from build123d import *

# Parameters (mm, degrees)
F1_DEPTH = 15
F3_DEPTH = 2.4
F4_R     = 1.8
F5_DEPTH = 13.301
F7_D     = 4


with BuildPart() as f1:
    # F0 (on Front) → F1 (new body)
    with BuildSketch(Plane.XZ):
        with BuildLine():
            Line((40, 0), (0, 0))
            Line((0, 0), (0, -3))
            Line((0, -3), (40, -3))
            ThreePointArc((40, -3), (47.202138, 7.972773), (34.269901, 10.215488))
            ThreePointArc((34.269901, 10.215488), (31.944896, 8.577711), (29.160258, 8))
            Line((29.160258, 8), (13, 8))
            Line((13, 8), (13, 5))
            Line((13, 5), (29.160258, 5))
            ThreePointArc((29.160258, 5), (33.138313, 5.825302), (36.459748, 8.164983))
            ThreePointArc((36.459748, 8.164983), (44.449729, 6.779356), (40, 0))
        make_face()
    extrude(amount=F1_DEPTH)

    # F2 (on face) → F3 (cut)
    with BuildSketch(Plane(origin=(0, 0, -3), x_dir=(1, 0, 0), z_dir=(0, 0, -1))):
        Polygon((21.645448, 10.35), (18.354552, 10.35), (16.709103, 7.5), (18.354552, 4.65), (21.645448, 4.65), (23.290897, 7.5), align=None)
    extrude(amount=-F3_DEPTH, mode=Mode.SUBTRACT)

    # F4 (on face) → F5 (cut, through all)
    with BuildSketch(Plane(origin=(0, 0, -0.6), x_dir=(1, 0, 0), z_dir=(0, 0, -1))):
        with Locations((20, 7.5)):
            Circle(F4_R)
    extrude(amount=-F5_DEPTH, mode=Mode.SUBTRACT)

    # F7 (through all)
    with Locations(Plane.XY):
        with Locations((7, -7.5)):
            Hole(F7_D / 2)


solid = f1.part
Design review of the part built by this model. Coordinates are the model's own, in mm. A direction names the side the tool comes from. Coordinates: 2 decimals unless noted, no trailing zeros. Write each loop counter-clockwise with the first axis right and the second up, starting at its lowest first coordinate (ties: lowest second). Pieces come first, ordered by that corner, then holes. Notation, with made-up numbers: (-17.5, 88) - (39.5, 88) arc R15 cw to (39.5, 103) - close; hole circle Ø2 at (-11, 28). An arc over 180 degrees is marked (long way). Use one line per item in the form item = value.
Q1. The part is to be moulded in two halves that separate along Z. For faces 1 (the flat face through (21, -5.7, 5)), 2 (the flat face through (20, -11, -3)), 3 (the flat face through (0, -7, -1)), 4 (the flat face through (21.2, -5.7, 8)), say which applies: +Z half, -Z half, draft (parallel to the pull), parting line (faces both ways), or undercut.
Taken from the geometry:
face_1 = undercut
face_2 = -Z half
face_3 = draft
face_4 = +Z half
Q2. Consider section D-D (y = -8.5). Write out the cut boundary in (x, z), plus the area to 3 significant figures.
Taken from the geometry:
outline = (0, -3) - (5.27, -3) - (5.27, 0) - (0, 0) - close; (8.73, -3) - (17.29, -3) - (17.29, -0.6) - (18.5, -0.6) - (18.5, 0) - (8.73, 0) - close; (13, 5) - (18.5, 5) - (18.5, 8) - (13, 8) - close; (21.5, -0.6) - (22.71, -0.6) - (22.71, -3) - (40, -3) arc R7.85 ccw (long way) to (34.27, 10.22) arc R7 cw to (29.16, 8) - (21.5, 8) - (21.5, 5) - (29.16, 5) arc R10 ccw to (36.46, 8.16) arc R4.85 cw (long way) to (40, 0) - (21.5, 0) - close
area = 231 mm^2
Q3. Insertion check: pin 1 Ø1 at (x, y) = (35, -11) entering from +Z; pin 2 Ø2.5 at (y, z) = (-5, 6.5) entering from -X; pin 3 Ø4.5 at (x, y) = (7, -7.5) entering from +Z. Each pin has a flat end and moves straight along its axis. Give the tip position at first contact, or say it passes through.
Taken from the geometry:
pin_1 = 11.28
pin_2 = 13
pin_3 = 0
Q4. For probe 1 along Z at (x, y) = (23, -6.5); probe 2 along Y at (x, z) = (7, -0.65); probe 3 along Y at (x, z) = (20, -0.4), list the stretches that pass through material, from the lowest coordinate up.
Taken from the geometry:
probe_1 = -3 to 0, 5 to 8
probe_2 = -15 to -9.5, -5.5 to 0
probe_3 = -15 to -9.3, -5.7 to 0
Q5. Machinability: for faces 5 (the flat face through (13, -7, 7)), 6 (the cylindrical face through (33.086, -7.395, 5.803)), 7 (the flat face through (22, -8, -0.6)), 8 (the flat face through (20, -11, 0)), which of the approach directions +Z, -Z, +X, -X, +Y, -Y give a long, thin tool a straight path to every point of the face, cutting with its end or side? Answer none if there is none.
Taken from the geometry:
face_5 = +Z, -X, +Y, -Y
face_6 = +Y, -Y
face_7 = -Z
face_8 = -X, +Y, -Y
Q6. Consider section B-B (y = -4). Write out the cut boundary in (x, z), plus the area to 3 significant figures.
Taken from the geometry:
outline = (0, -3) - (40, -3) arc R7.85 ccw (long way) to (34.27, 10.22) arc R7 cw to (29.16, 8) - (13, 8) - (13, 5) - (29.16, 5) arc R10 ccw to (36.46, 8.16) arc R4.85 cw (long way) to (40, 0) - (0, 0) - close
area = 265 mm^2
Q7. Consider section A-A (x = 25). Write out the cut boundary in (y, z), plus the area to 3 significant figures.
Taken from the geometry:
outline = (-15, -3) - (0, -3) - (0, 0) - (-15, 0) - close; (-15, 5) - (0, 5) - (0, 8) - (-15, 8) - close
area = 90.0 mm^2
Q8. Consider section C-C (x = 20). Write out the cut boundary in (y, z).
Taken from the geometry:
outline = (-15, -3) - (-10.35, -3) - (-10.35, -0.6) - (-9.3, -0.6) - (-9.3, 0) - (-15, 0) - close; (-15, 5) - (-9.3, 5) - (-9.3, 8) - (-15, 8) - close; (-5.7, -0.6) - (-4.65, -0.6) - (-4.65, -3) - (0, -3) - (0, 0) - (-5.7, 0) - close; (-5.7, 5) - (0, 5) - (0, 8) - (-5.7, 8) - close
